Could you check a few things on this model? Use its own coordinates, in mm. Round coordinates to 2 decimals unless told otherwise and drop trailing zeros. Write each loop counter-clockwise with the first axis right and the second up, starting at its lowest first coordinate (ties: lowest second). Pieces come first, ordered by that corner, then holes. Notation, with made-up numbers: (75.25, 24.25) -> (104.25, 24.25) arc R9 ccw to (104.25, 29.25) -> close; hole circle Ø5 at (32, 48.5). An arc over 180 degrees is marked (long way). Answer in a Markdown table with one row per item.
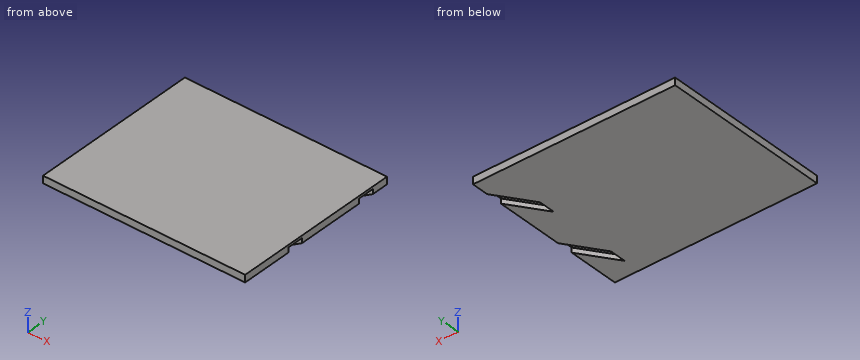
from build123d import *

# Parameters (mm, degrees)
F1_DEPTH = 70
F3_DEPTH = 2


# Not quite as in the source:
# - a feature names something its author has since deleted; it is built from what else it names


with BuildPart() as f1:
    # F0 (on Front) → F1 (new body)
    with BuildSketch(Plane.XZ):
        Polygon((0, -20), (0, -23), (32, -23), (32, -21), (38, -21), (42, -21), (42, -20), align=None)
        Polygon((-32, -23), (0, -23), (0, -20), (-17, -20), (-21, -20), (-30, -20), (-34, -20), (-34, -21), (-32, -21), align=None)
        Polygon((32, -21), (32, -23), (38, -23), (38, -22.25), (38, -21), align=None)
        Polygon((-38, -23), (-32, -23), (-32, -21), (-34, -21), (-38, -21), (-38, -22.25), align=None)
        Polygon((38, -22.25), (38, -23), (42, -23), (42, -21), (38, -21), align=None)
        Polygon((-42, -23), (-38, -23), (-38, -22.25), (-38, -21), (-42, -21), align=None)
        Polygon((-38, -21), (-34, -21), (-34, -20), (-42, -20), (-42, -21), align=None)
    extrude(amount=F1_DEPTH)

    # F2 (on face) → F3 (cut)
    with BuildSketch(Plane(origin=(0, 0, -23), x_dir=(1, 0, 0), z_dir=(0, 0, -1))):
        Polygon((42, 42), (42, 48.7185199326), (32, 63), (32, 56.2814800674), align=None)
        Polygon((42, 7), (42, 13.7185199326), (32, 28), (32, 21.2814800674), align=None)
    extrude(amount=-F3_DEPTH, mode=Mode.SUBTRACT)


solid = f1.part
1) Imagine slicing it at D-D, the plane y = -12. Please give me the cut outline in (x, z), plus the area to 3 significant figures.
Findings:
| item | result |
|---|---|
| outline | (-42, -23) -> (38.5, -23) -> (38.5, -21) -> (42, -21) -> (42, -20) -> (-42, -20) -> close |
| area | 245 mm^2 |
2) Imagine slicing it at A-A, the plane y = -53.5. Please give me the cut outline in (x, z).
Findings:
| item | result |
|---|---|
| outline | (-42, -23) -> (33.95, -23) -> (33.95, -21) -> (38.65, -21) -> (38.65, -23) -> (42, -23) -> (42, -20) -> (-42, -20) -> close |
3) Imagine slicing it at C-C, the plane x = 37. Please give me the cut outline in (y, z), plus the area to 3 significant figures.
Findings:
| item | result |
|---|---|
| outline | (-70, -23) -> (-55.86, -23) -> (-55.86, -21) -> (-49.14, -21) -> (-49.14, -23) -> (-20.86, -23) -> (-20.86, -21) -> (-14.14, -21) -> (-14.14, -23) -> (0, -23) -> (0, -20) -> (-70, -20) -> close |
| area | 183 mm^2 |
4) Please list where these lines run through material, in increasing order: line 1 (X direction, y = -21, z = -21.8); line 2 (X direction, y = -20, z = -21.55).
Findings:
| item | result |
|---|---|
| line 1 | x = -42 to 32.2, 36.9 to 42 |
| line 2 | x = -42 to 32.9, 37.6 to 42 |
5) Imagine slicing it at B-B, the plane z = -22.3. Please give me the cut outline in (x, y).
Findings:
| item | result |
|---|---|
| outline | (-42, -70) -> (42, -70) -> (42, -48.72) -> (32, -63) -> (32, -56.28) -> (42, -42) -> (42, -13.72) -> (32, -28) -> (32, -21.28) -> (42, -7) -> (42, 0) -> (-42, 0) -> close |
